Could you check a few things on this drawing? It's one solid part, dimensions in mm from its lowest x, y, z. Give positions to 0.01 mm unless a question says otherwise; leave off trailing zeros. Write each loop counter-clockwise with the first axis right and the second up, starting at its lowest first coordinate (ties: lowest second). Pieces come first, ordered by that corner, then holes. Notation, with made-up numbers: (19, 83) -> (74, 83) arc R23 cw to (74, 97) -> close; hole circle Ø2 at (45.5, 10). An arc over 180 degrees is marked (long way). Use CSV: the item, a comma, the result in double quotes. Start each with the question number.
(1) Suppose I cut it at B-B on z = 50. List the corners of the cut face in (x, y) for me.
(2) Suppose I cut it at C-C on x = 12. List the corners of the cut face in (y, z) for me.
(3) For pin 1 Ø4 at (x, z) = (50, 12) entering from -Y; pin 2 Ø3 at (x, y) = (39, 4.5) entering from +Z; pin 3 Ø1 at (y, z) = (2, 20.5) entering from +X, each with a flat end and sliding along its axis, tell me the tip position at first contact or that it passes through.
(4) Suppose I cut it at D-D on x = 22. List the corners of the cut face in (y, z) for me.
(5) I need wall thicknesses on L1, parallel to Z at x = 50, y = 4.4; L2, parallel to X at y = 1.05, z = 33; L3, parallel to X at y = 1.05, z = 52. Which ranges of each line are inside material? Lowest first, please. Write a range as [from, to].
(6) Suppose I cut it at A-A on y = 4.05. List the corners of the cut face in (x, z) for me, plus the area to 3 significant figures.
(7) If we mould it in two halves opening along X, with no side actions, what happens to the marked faces 1, 2 and 3? For each: pulls with the +X half, pulls with the -X half, needs draft (parallel to the pull), parting line crosses it, or undercut.
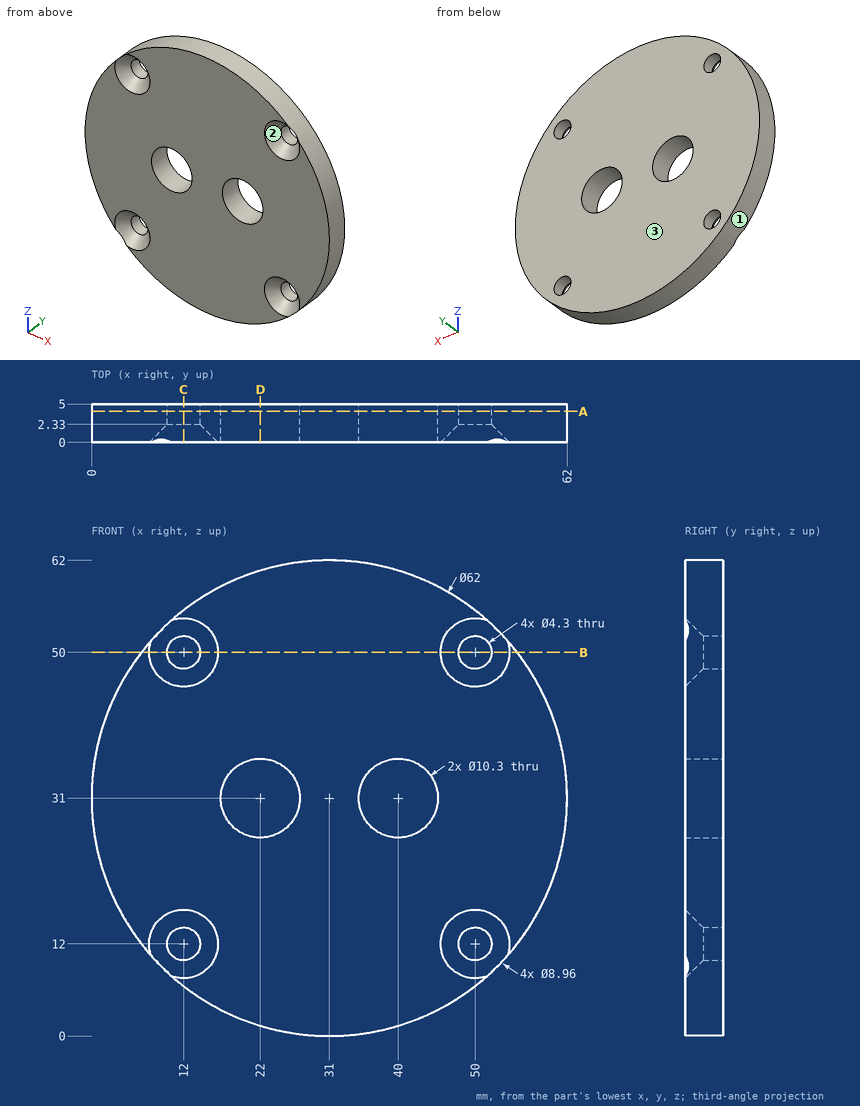
Geometry says:
1,outline,"(6.51, 0) -> (7.52, 0) -> (9.85, 2.33) -> (9.85, 5) -> (6.51, 5) -> close; (14.15, 2.33) -> (16.48, 0) -> (45.52, 0) -> (47.85, 2.33) -> (47.85, 5) -> (14.15, 5) -> close; (52.15, 2.33) -> (54.48, 0) -> (55.49, 0) -> (55.49, 5) -> (52.15, 5) -> close"
2,outline,"(0, 6.51) -> (5, 6.51) -> (5, 9.85) -> (2.33, 9.85) -> (0, 7.52) -> close; (0, 16.48) -> (2.33, 14.15) -> (5, 14.15) -> (5, 47.85) -> (2.33, 47.85) -> (0, 45.52) -> close; (0, 54.48) -> (2.33, 52.15) -> (5, 52.15) -> (5, 55.49) -> (0, 55.49) -> close"
3,pin 1,"through"
3,pin 2,"z = 61.31"
3,pin 3,"x = 60.34"
4,outline,"(0, 1.34) -> (5, 1.34) -> (5, 25.85) -> (0, 25.85) -> close; (0, 36.15) -> (5, 36.15) -> (5, 60.66) -> (0, 60.66) -> close"
5,L1,"[6.51, 9.85], [14.15, 47.85], [52.15, 55.49]"
5,L2,"[0.06, 17.25], [26.75, 35.25], [44.75, 61.94]"
5,L3,"[8.2, 9.21], [14.79, 47.21], [52.79, 53.8]"
6,outline,"circle Ø62 at (31, 31); hole circle Ø4.3 at (12, 12); hole circle Ø4.3 at (12, 50); hole circle Ø10.3 at (22, 31); hole circle Ø10.3 at (40, 31); hole circle Ø4.3 at (50, 12); hole circle Ø4.3 at (50, 50)"
6,area,"2,790 mm²"
7,face 1,"parting line crosses it"
7,face 2,"undercut"
7,face 3,"needs draft"
